from build123d import *

# Parameters (mm, degrees)
SKETCH1_W           = 35
SKETCH1_H           = 50
BOSS_EXTRUDE1_DEPTH = 5
SKETCH2_R           = 1.75
CUT_EXTRUDE1_DEPTH  = 6
SKETCH3_W           = 12.5
SKETCH3_H           = 5
BOSS_EXTRUDE2_DEPTH = 40
SKETCH4_W           = 10
SKETCH4_H           = 5
BOSS_EXTRUDE3_DEPTH = 24
SKETCH5_R           = 1.75
CUT_EXTRUDE2_DEPTH  = 36


with BuildPart() as part:
    # Sketch1 → Boss-Extrude1 (new body)
    with BuildSketch(Plane(origin=(0, 0, 0), x_dir=(1, 0, 0), z_dir=(0, 1, 0))):
        with Locations((17.5, 25)):
            Rectangle(SKETCH1_W, SKETCH1_H)
    extrude(amount=BOSS_EXTRUDE1_DEPTH)

    # Sketch2 → Cut-Extrude1 (cut, through all)
    with BuildSketch(Plane(origin=(0, 5, 0), x_dir=(1, 0, 0), z_dir=(0, 1, 0))):
        with Locations((9.75, 11.75)):
            Circle(SKETCH2_R)
        with Locations((9.75, 25.25)):
            Circle(SKETCH2_R)
        with Locations((25.25, 11.75)):
            Circle(SKETCH2_R)
        with Locations((25.25, 25.25)):
            Circle(SKETCH2_R)
    extrude(amount=-CUT_EXTRUDE1_DEPTH, mode=Mode.SUBTRACT)

    # Sketch3 → Boss-Extrude2 (add)
    with BuildSketch(Plane(origin=(0, 5, 0), x_dir=(1, 0, 0), z_dir=(0, 1, 0))):
        with Locations((6.25, 47.5)):
            Rectangle(SKETCH3_W, SKETCH3_H)
        with Locations((28.75, 47.5)):
            Rectangle(SKETCH3_W, SKETCH3_H)
    extrude(amount=BOSS_EXTRUDE2_DEPTH)

    # Sketch4 → Boss-Extrude3 (add)
    with BuildSketch(Plane(origin=(0, 5, 0), x_dir=(1, 0, 0), z_dir=(0, 1, 0))):
        with Locations((17.5, 47.5)):
            Rectangle(SKETCH4_W, SKETCH4_H)
    extrude(amount=BOSS_EXTRUDE3_DEPTH)

    # Sketch5 → Cut-Extrude2 (cut, through all)
    with BuildSketch(Plane.ZY):
        with Locations((-47.5, 41.5)):
            Circle(SKETCH5_R)
    extrude(amount=-CUT_EXTRUDE2_DEPTH, mode=Mode.SUBTRACT)


solid = part.part
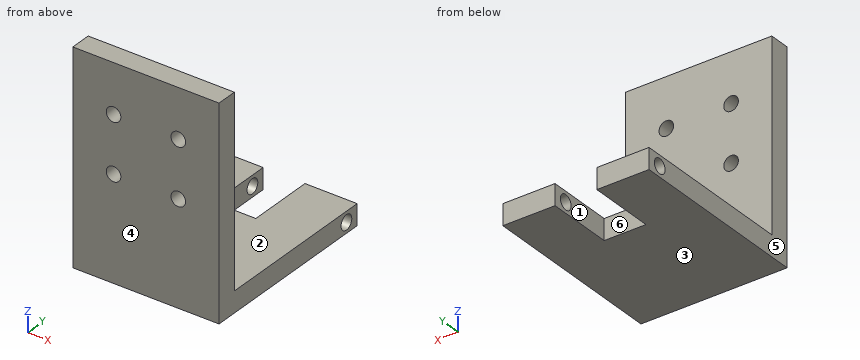
The model under review builds one solid part; all positions refer to its coordinate system, in mm. Face numbers are marked on the shaded views. A direction names the side the tool comes from. Coordinates: 2 decimals unless noted, no trailing zeros. Loops run counter-clockwise (first coordinate to the right, second up) from the corner with the lowest first, then second, coordinate; pieces in that order, holes last.
(1) Tool access review of the marked faces 1, 2 and 3: name each direction out of +Z, -Z, +X, -X, +Y, -Y from which nothing blocks a thin tool from reaching the whole face with its end or side.
Determined:
face 1: +Z, -Z, +Y
face 2: +Z, +X, -X, +Y
face 3: -Z, +X, -X, +Y, -Y
(2) Draft analysis for pull direction X (two halves, no side actions). For the marked faces 4, 5 and 6, state which applies: +X half, -X half, draft (parallel to the pull), parting line (faces both ways), or undercut.
Determined:
face 4: draft
face 5: -X half
face 6: undercut
(3) Consider section C-C, the plane y = 41.5. Give the boundary of the cut face in (x, z).
Determined:
outline: (0, -50) - (12.5, -50) - (12.5, -49.25) - (0, -49.25) - close; (0, -45.75) - (12.5, -45.75) - (12.5, -45) - (0, -45) - close; (22.5, -50) - (35, -50) - (35, -49.25) - (22.5, -49.25) - close; (22.5, -45.75) - (35, -45.75) - (35, -45) - (22.5, -45) - close
(4) Consider section D-D, the plane y = 36.5. Give the boundary of the cut face in (x, z), plus the area to 3 significant figures.
Determined:
outline: (0, -50) - (12.5, -50) - (12.5, -45) - (0, -45) - close; (22.5, -50) - (35, -50) - (35, -45) - (22.5, -45) - close
area: 125 mm2
(5) Consider section B-B, the plane x = 25.25. Give the boundary of the cut face in (y, z), plus the area to 3 significant figures.
Determined:
outline: (0, -50) - (45, -50) - (45, -45) - (5, -45) - (5, -27) - (0, -27) - close; (0, -23.5) - (5, -23.5) - (5, -13.5) - (0, -13.5) - close; (0, -10) - (5, -10) - (5, 0) - (0, 0) - close; hole circle Ø3.5 at (41.5, -47.5)
area: 405 mm2
(6) Insertion check: P1, Ø2.5, axis at x = 16.5, z = -48, coming from the +Y side; P2, Ø17.5, axis at x = 17.5, z = -30.5, coming from the +Y side. Each pin has a flat end and moves straight along its axis. Give the tip position at first contact, or say it passes through.
Determined:
P1: stops at y = 29
P2: stops at y = 5
(7) Consider section A-A, the plane z = -11.75. Give the boundary of the cut face in (x, y).
Determined:
outline: (0, 0) - (8, 0) - (8, 5) - (0, 5) - close; (11.5, 0) - (23.5, 0) - (23.5, 5) - (11.5, 5) - close; (27, 0) - (35, 0) - (35, 5) - (27, 5) - close
(8) Wall thickness on L1, parallel to Z at x = 25.25, y = 2.4; L2, parallel to X at y = 2.6, z = -25.25; L3, parallel to Y at x = 27.5, z = -47.5: over which ranges is each line inside the solid? List them lowest first.
Determined:
L1: z = -50 to -27, -23.5 to -13.5, -10 to 0
L2: x = 0 to 8, 11.5 to 23.5, 27 to 35
L3: y = 0 to 39.75, 43.25 to 45
